Model file for the job. Use its own axes, mm. Face numbers are marked on the shaded views. Give positions to 0.01 mm unless a question says otherwise; leave off trailing zeros. Write each loop counter-clockwise with the first axis right and the second up, starting at its lowest first coordinate (ties: lowest second). Pieces come first, ordered by that corner, then holes.
```python
from build123d import *

# Parameters (mm, degrees)
SKETCH2_R           = 50
BOSS_EXTRUDE1_DEPTH = 25
FILLET1_R           = 2.5
SKETCH3_R           = 6
CUT_EXTRUDE1_DEPTH  = 25


with BuildPart() as part:
    # Sketch2 → Boss-Extrude1 (new body)
    with BuildSketch(Plane(origin=(0, 0, 0), x_dir=(0, 0, -1), z_dir=(1, 0, 0))):
        Circle(SKETCH2_R)
    extrude(amount=-BOSS_EXTRUDE1_DEPTH)

    # Fillet1
    fillet1_edges = [part.edges().sort_by_distance(p)[0] for p in [
        (0, 0, 50),
        (-25, 0, 50),
    ]]
    fillet(fillet1_edges, radius=FILLET1_R)

    # Sketch3 → Cut-Extrude1 (cut)
    with BuildSketch(Plane.ZY.offset(25)):
        Circle(SKETCH3_R)
    extrude(amount=-CUT_EXTRUDE1_DEPTH, mode=Mode.SUBTRACT)


solid = part.part
```
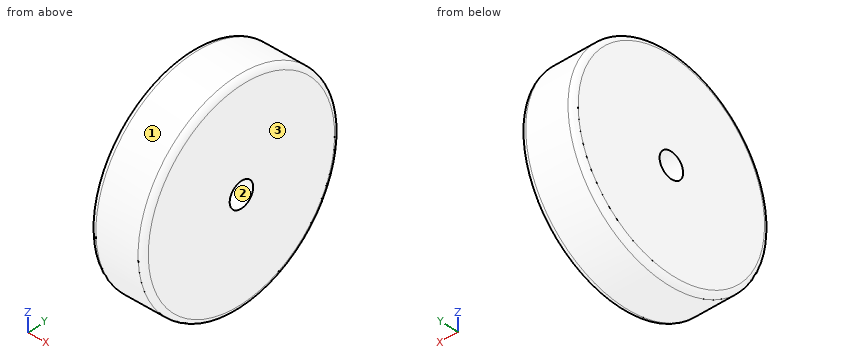
1. Pull direction Z, two halves, no side cores. Call the marked faces 1, 2 and 3: +Z half, -Z half, draft (parallel to the pull), parting line (faces both ways), or undercut.
Calculated:
face 1: parting line
face 2: undercut
face 3: draft
2. Slice it at C-C, the plane x = -11. Write the cut outline in (y, z), and give its area (3 significant figures).
Calculated:
outline: circle Ø100 at (0, 0); hole circle Ø12 at (0, 0)
area: 7,740 mm2
3. Slice it at A-A, the plane z = 0. Write the cut outline in (x, y).
Calculated:
outline: (-25, -47.5) arc R2.5 ccw to (-22.5, -50) - (-2.5, -50) arc R2.5 ccw to (0, -47.5) - (0, -6) - (-25, -6) - close; (-25, 6) - (0, 6) - (0, 47.5) arc R2.5 ccw to (-2.5, 50) - (-22.5, 50) arc R2.5 ccw to (-25, 47.5) - close
4. Probe probe 1 along Y at (x, z) = (-14.75, 0); probe 2 along Y at (x, z) = (-11, -17.5); probe 3 along Y at (x, z) = (-11.75, 20). List the from-to ranges inside material, lowest first.
Calculated:
probe 1: y = -50 to -6, 6 to 50
probe 2: y = -46.84 to 46.84
probe 3: y = -45.83 to 45.83
5. Pin check, flat tips, straight feed: P1, Ø4, axis at x = -5, y = 39.5, coming from the -Z side; P2, Ø3, axis at x = -16.5, z = -31.5, coming from the +Y side; P3, Ø12, axis at x = -19.5, z = 35, coming from the +Y side. Stop position of each tip, or through.
Calculated:
P1: stops at z = -33.07
P2: stops at y = 40
P3: stops at y = 40.73
